Read the model definition and answer for the solid it produces. Units are mm, in the model's axes. A direction names the side the tool comes from. Round coordinates to 2 decimals unless told otherwise and drop trailing zeros. Order: outer loops, then holes, each group sorted by start corner. A loop starts at its lowest first (then second) coordinate and runs counter-clockwise, first axis right, second up. Notation, with made-up numbers: (89.25, 10) - (121.25, 10) arc R23 ccw to (121.25, 36) - close; hole circle Ø8 at (75.5, -24.75). An arc over 180 degrees is marked (long way). Answer as a JSON object with one key per item and string values. Group by question number.
Q1. A tool of negligible diameter and unlimited length cuts with its end or side. For faces 1 (the flat face through (-314.418, 199, 3)), 2 (the flat face through (-313.548, 268, 3)), from which of +Z, -Z, +X, -X, +Y, -Y can it reach the whole face along a straight path? Write none if from no direction.
Q2. Given pin 1 Ø3 at (x, z) = (-337, 2) entering from -Y; pin 2 Ø3 at (y, z) = (263, 4.5) entering from -X; pin 3 Ø8 at (x, y) = (-339, 306.5) entering from -Z, each flat-ended and moving along its own axis, determine where each tip first touches the part or whether it passes through.
Q3. A cutting plane is placed at B-B on x = -331.5. Determine the outline of the cut face in (y, z).
Q4. A cutting plane is placed at A-A on x = -319.5. Determine the outline of the cut face in (y, z).
Q5. A cutting plane is placed at C-C on z = 1.75. Count the separate pieces of the cut face and the enclosed holes in it, and give its area (3 significant figures).
Q6. Consider line 1 (Y direction, x = -322.5, z = 5.5); line 2 (Y direction, x = -325.5, z = 2.25); line 3 (X direction, y = 194.5, z = 5.75). Determine where each line is inside the solid, lowest interval first.
Q7. The mould has two halves that part along X. Classify faces 3 (the flat face through (-311, 135.786, 3)), 4 (the flat face through (-319, 251.33, 3)), 5 (the flat face through (-342.708, 230, 3)): pulls with the +X half, pulls with the -X half, needs draft (parallel to the pull), parting line crosses it, or undercut.
```python
from build123d import *

# Parameters (mm, degrees)
SKETCH2_W           = 40.132
SKETCH2_H           = 190.436
BOSS_EXTRUDE1_DEPTH = 6.35
SKETCH3_R           = 3.3
CUT_EXTRUDE1_DEPTH  = 478.183864302
SKETCH4_W           = 10.033
SKETCH4_H           = 6.858
CUT_EXTRUDE2_DEPTH  = 474.191260281


with BuildPart() as part:
    # Sketch2 → Boss-Extrude1 (new body)
    with BuildSketch(Plane.XY):
        with Locations((-328.134441571, 231.003658294)):
            Rectangle(SKETCH2_W, SKETCH2_H)
    extrude(amount=BOSS_EXTRUDE1_DEPTH)

    # Sketch3 → Cut-Extrude1 (cut, through all)
    with BuildSketch(Plane.XY.offset(6.35)):
        Polygon((-314.418441571, 195.840658294), (-314.418441571, 203.079658294), (-342.708441633, 203.079658294), (-342.708441633, 257.927658294), (-314.418441571, 257.927658294), (-314.418441571, 265.166658294), (-342.708441633, 265.166658294), (-342.708441633, 321.014658294), (-314.418441571, 321.014658294), (-314.418441571, 326.221658294), (-348.200441571, 326.221658294), (-348.200441571, 135.785658294), (-314.418441571, 135.785658294), (-314.418441571, 140.992658294), (-342.708441633, 140.992658294), (-342.708441633, 195.840658294), align=None)
        with Locations((-332.325441571, 294.535658294)):
            Circle(SKETCH3_R)
        with Locations((-332.325441571, 231.035658294)):
            Circle(SKETCH3_R)
        with Locations((-332.325441571, 167.535658294)):
            Circle(SKETCH3_R)
    extrude(amount=-CUT_EXTRUDE1_DEPTH, mode=Mode.SUBTRACT)

    # Sketch4 → Cut-Extrude2 (cut, through all)
    with BuildSketch(Plane.XY.offset(6.35)):
        with Locations((-318.564971808, 144.167658294)):
            Rectangle(SKETCH4_W, SKETCH4_H)
        with Locations((-318.564971808, 192.656258294)):
            Rectangle(SKETCH4_W, SKETCH4_H)
        with Locations((-318.564971808, 206.245258294)):
            Rectangle(SKETCH4_W, SKETCH4_H)
        with Locations((-318.564971808, 254.759258294)):
            Rectangle(SKETCH4_W, SKETCH4_H)
        with Locations((-318.564971808, 268.348258294)):
            Rectangle(SKETCH4_W, SKETCH4_H)
        with Locations((-318.564971808, 317.852858294)):
            Rectangle(SKETCH4_W, SKETCH4_H)
    extrude(amount=-CUT_EXTRUDE2_DEPTH, mode=Mode.SUBTRACT)


solid = part.part
```
Result set:
{
 "1": {"face 1": "+Z, -Z, -X", "face 2": "+Z, -Z"},
 "2": {"pin 1": "stops at y = 140.99", "pin 2": "stops at x = -314.42", "pin 3": "stops at z = 0"},
 "3": {"outline": "(140.99, 0) - (164.34, 0) - (164.34, 6.35) - (140.99, 6.35) - close; (170.73, 0) - (195.84, 0) - (195.84, 6.35) - (170.73, 6.35) - close; (203.08, 0) - (227.84, 0) - (227.84, 6.35) - (203.08, 6.35) - close; (234.23, 0) - (257.93, 0) - (257.93, 6.35) - (234.23, 6.35) - close; (265.17, 0) - (291.34, 0) - (291.34, 6.35) - (265.17, 6.35) - close; (297.73, 0) - (321.01, 0) - (321.01, 6.35) - (297.73, 6.35) - close"},
 "4": {"outline": "(147.6, 0) - (189.23, 0) - (189.23, 6.35) - (147.6, 6.35) - close; (209.67, 0) - (251.33, 0) - (251.33, 6.35) - (209.67, 6.35) - close; (271.78, 0) - (314.42, 0) - (314.42, 6.35) - (271.78, 6.35) - close"},
 "5": {"separate pieces": "1", "enclosed holes": "3", "area": "5,390 mm²"},
 "6": {"line 1": "y = 147.6 to 189.23, 209.67 to 251.33, 271.78 to 314.42", "line 2": "y = 140.99 to 195.84, 203.08 to 257.93, 265.17 to 321.01", "line 3": "x = -342.71 to -323.58, -313.55 to -308.07"},
 "7": {"face 3": "needs draft", "face 4": "undercut", "face 5": "pulls with the -X half"}
}
